from build123d import *

# Parameters (mm, degrees)
BOSS_EXTRUDE1_DEPTH      = 76.2
SKETCH2_W                = 6.985
SKETCH2_H                = 9.525
CUT_EXTRUDE1_DEPTH       = 119.84173867
CUT_EXTRUDE2_DEPTH       = 119.84173867
CUT_EXTRUDE3_DEPTH       = 119.84173867
FILLET1_R                = 2.54
CUT_EXTRUDE4_DEPTH       = 5.08
CUT_EXTRUDE6_DEPTH       = 15.113
FILLET2_R                = 0.508
BOSS_EXTRUDE3_DEPTH      = 31.115
BOSS_EXTRUDE4_DEPTH      = 5.08
CUT_EXTRUDE7_DEPTH       = 85.888967529
CRVPATTERN3_START        = 20.1179377
CRVPATTERN3_OUTLINE_W    = 31.115
CRVPATTERN3_OUTLINE_H    = 7.094089262
CRVPATTERN3_DEPTH        = 4.784345088
CRVPATTERN3_START_2      = 12.248105014
CRVPATTERN3_2_OUTLINE_W  = 31.115
CRVPATTERN3_2_OUTLINE_H  = 6.763167552
CRVPATTERN3_2_DEPTH      = 4.784345087
CRVPATTERN3_START_3      = 4.095774155
CRVPATTERN3_3_OUTLINE_W  = 31.115
CRVPATTERN3_3_OUTLINE_H  = 6.419828923
CRVPATTERN3_3_DEPTH      = 4.784345087
CRVPATTERN3_START_4      = -4.324087509
CRVPATTERN3_4_OUTLINE_W  = 31.115
CRVPATTERN3_4_OUTLINE_H  = 6.064703736
CRVPATTERN3_4_DEPTH      = 4.784345087
CRVPATTERN3_START_5      = 27.690823503
CRVPATTERN3_5_OUTLINE_W  = 31.115
CRVPATTERN3_5_OUTLINE_H  = 6.047255266
CRVPATTERN3_5_DEPTH      = 4.784345088
CRVPATTERN3_START_6      = -12.996021434
CRVPATTERN3_6_OUTLINE_W  = 31.115
CRVPATTERN3_6_OUTLINE_H  = 5.698443985
CRVPATTERN3_6_DEPTH      = 4.784345087
CRVPATTERN3_START_7      = -21.904106282
CRVPATTERN3_7_OUTLINE_W  = 31.115
CRVPATTERN3_7_OUTLINE_H  = 5.321722107
CRVPATTERN3_7_DEPTH      = 4.784345088
CRVPATTERN3_START_8      = -31.031987149
CRVPATTERN3_8_OUTLINE_W  = 31.115
CRVPATTERN3_8_OUTLINE_H  = 4.935229754
CRVPATTERN3_8_DEPTH      = 4.784345087
CRVPATTERN3_START_9      = -40.362905596
CRVPATTERN3_9_OUTLINE_W  = 31.115
CRVPATTERN3_9_OUTLINE_H  = 4.539676505
CRVPATTERN3_9_DEPTH      = 4.784345087
CRVPATTERN3_START_10     = -49.879730415
CRVPATTERN3_10_OUTLINE_W = 31.115
CRVPATTERN3_10_OUTLINE_H = 4.135788586
CRVPATTERN3_10_DEPTH     = 4.784345088
CRVPATTERN3_START_11     = -59.564989077
CRVPATTERN3_11_OUTLINE_W = 31.115
CRVPATTERN3_11_OUTLINE_H = 3.724307516
CRVPATTERN3_11_DEPTH     = 4.784345087
FILLET3_R                = 5.08


# Read off the part's stored shape, not the designer's step: CrvPattern3
with BuildPart() as part:
    # Sketch1 → Boss-Extrude1 (new body)
    with BuildSketch(Plane.XY):
        Polygon((-15.5575, 76.2), (15.5575, 76.2), (15.5575, -76.2), (7.845485509, -76.2), (9.525, -85.725), (-9.525, -85.725), (-7.845485509, -76.2), (-15.5575, -76.2), align=None)
    extrude(amount=BOSS_EXTRUDE1_DEPTH)

    # Sketch2 → Cut-Extrude1 (cut, through all)
    with BuildSketch(Plane(origin=(15.5575, 0, 0), x_dir=(0, 0, -1), z_dir=(1, 0, 0))):
        with Locations((-3.4925, -80.9625)):
            Rectangle(SKETCH2_W, SKETCH2_H)
    extrude(amount=-CUT_EXTRUDE1_DEPTH, mode=Mode.SUBTRACT)

    # Sketch3 → Cut-Extrude2 (cut, through all)
    with BuildSketch(Plane(origin=(15.5575, 0, 0), x_dir=(0, 0, -1), z_dir=(1, 0, 0))):
        with BuildLine():
            Line((-76.2, -85.725), (-76.2, -76.2))
            Line((-76.2, -76.2), (-76.2, 76.2))
            Line((-76.2, 76.2), (-6.541803462, 76.2))
            ThreePointArc((-6.541803462, 76.2), (-58.046669251, 2.411215556), (-76.2, -85.725))
        make_face()
        with BuildLine():
            Line((0, -76.2), (0, 67.75939176))
            ThreePointArc((0, 67.75939176), (-18.20597202, -4.22030412), (0, -76.2))
        make_face()
    extrude(amount=-CUT_EXTRUDE2_DEPTH, mode=Mode.SUBTRACT)

    # Sketch6 → Cut-Extrude3 (cut, through all)
    with BuildSketch(Plane(origin=(15.5575, 0, 0), x_dir=(0, 0, -1), z_dir=(1, 0, 0))):
        with BuildLine():
            ThreePointArc((-28.934409948, -61.883434575), (-23.879909813, -60.517759582), (-22.716254779, -55.412963136))
            ThreePointArc((-22.716254779, -55.412963136), (-30.753414225, -11.294498854), (-26.546552055, 33.352305435))
            ThreePointArc((-26.546552055, 33.352305435), (-49.181053892, -9.446405872), (-61.429710833, -56.286781256))
            ThreePointArc((-61.429710833, -56.286781256), (-59.737369376, -60.827463042), (-55.008021131, -61.883434575))
            ThreePointArc((-55.008021131, -61.883434575), (-41.971215539, -60.062859411), (-28.934409948, -61.883434575))
        make_face()
    extrude(amount=-CUT_EXTRUDE3_DEPTH, mode=Mode.SUBTRACT)

    # Fillet1
    fillet1_edges = [part.edges().sort_by_distance(p)[0] for p in [
        (0, 33.352305435, 26.546552055),
    ]]
    fillet(fillet1_edges, radius=FILLET1_R)

    # Sketch7 → Cut-Extrude4 (cut, symmetric)
    with BuildSketch(Plane(origin=(0, 0, 0), x_dir=(0, 0, -1), z_dir=(1, 0, 0))):
        with BuildLine():
            Line((-30.699128799, 4.016230293), (-17.981752538, 4.016230293))
            ThreePointArc((-17.981752538, 4.016230293), (-17.415803594, -19.667907964), (-13.161921654, -42.973769707))
            Line((-13.161921654, -42.973769707), (-26.264177108, -42.973769707))
            ThreePointArc((-26.264177108, -42.973769707), (-30.179968378, -19.639057999), (-30.699128799, 4.016230293))
        make_face()
    extrude(amount=CUT_EXTRUDE4_DEPTH, both=True, mode=Mode.SUBTRACT)

    # Sketch10 → Cut-Extrude6 (cut, symmetric)
    with BuildSketch(Plane(origin=(15.5575, 76.2, 6.541803462), x_dir=(-1, 0, 0), z_dir=(0, -0.7903999954772005, -0.6125910929401777))):
        Polygon((0, 5.170641427), (6.985, 5.170641427), (0, -3.655858573), align=None)
        Polygon((31.115, 5.170641427), (31.115, -3.655858573), (24.13, 5.170641427), align=None)
    extrude(amount=CUT_EXTRUDE6_DEPTH, both=True, mode=Mode.SUBTRACT)

    # Fillet2
    fillet2_edges = [part.edges().sort_by_distance(p)[0] for p in [
        (0, 76.2, 6.541803462),
        (-14.111333502, 74.930435776, 7.871138317),
        (14.111333502, 74.930435776, 7.871138317),
        (-15.5575, 5.090891194, 56.873019023),
        (15.5575, 5.090891194, 56.873019023),
    ]]
    fillet(fillet2_edges, radius=FILLET2_R)


with BuildPart() as body_2:
    # Sketch11 → Boss-Extrude3 (new body)
    with BuildSketch(Plane(origin=(15.5575, 0, 0), x_dir=(0, 0, -1), z_dir=(1, 0, 0))):
        with BuildLine():
            Line((-8.76443151, 48.407010808), (-3.38019913, 48.407010808))
            ThreePointArc((-3.38019913, 48.407010808), (-7.998658724, -12.530018981), (2.784381833, -72.682972398))
            Line((2.784381833, -72.682972398), (-1.84156903, -72.682972398))
            ThreePointArc((-1.84156903, -72.682972398), (-17.95915827, -12.861548832), (-8.76443151, 48.407010808))
        make_face()
    extrude(amount=-BOSS_EXTRUDE3_DEPTH)


with BuildPart() as body_3:
    # Sketch13 → Boss-Extrude4 (new, symmetric)
    with BuildSketch(Plane(origin=(0, 0, 0), x_dir=(0, 0, -1), z_dir=(1, 0, 0))):
        with BuildLine():
            Line((-13.161921654, -42.973769707), (-26.264177108, -42.973769707))
            ThreePointArc((-26.264177108, -42.973769707), (-30.179968378, -19.639057999), (-30.699128799, 4.016230293))
            Line((-30.699128799, 4.016230293), (-17.981752538, 4.016230293))
            ThreePointArc((-17.981752538, 4.016230293), (-17.415803594, -19.667907964), (-13.161921654, -42.973769707))
        make_face()
    extrude(amount=BOSS_EXTRUDE4_DEPTH, both=True)


with BuildPart() as body_2_1:
    add(body_2.part)

    # Combine1: union body 3
    add(body_3.part)

    # Sketch14 → Cut-Extrude7 (cut, through all)
    with BuildSketch(Plane(origin=(15.5575, 0, 0), x_dir=(0, 0, -1), z_dir=(1, 0, 0))):
        Polygon((-3.636956276, 47.137010808), (-0.743194378, 43.327010808), (-4.923479567, 40.152010808), (-7.817241465, 43.962010808), align=None)
    extrude(amount=-CUT_EXTRUDE7_DEPTH, mode=Mode.SUBTRACT)

    # CrvPattern3 outline → CrvPattern3 (cut)
    with BuildSketch(Plane(origin=(0, 0, 0), x_dir=(1, 0, 0), z_dir=(0, 0.7963472387815729, 0.604839710406786)).offset(CRVPATTERN3_START)):
        with Locations((0, 9.405700103)):
            Rectangle(CRVPATTERN3_OUTLINE_W, CRVPATTERN3_OUTLINE_H)
    extrude(amount=CRVPATTERN3_DEPTH, mode=Mode.SUBTRACT)

    # CrvPattern3 2 outline → CrvPattern3 2 (cut)
    with BuildSketch(Plane(origin=(0, 0, 0), x_dir=(1, 0, 0), z_dir=(0, 0.7963472387815729, 0.604839710406786)).offset(CRVPATTERN3_START_2)):
        with Locations((0, 2.477071696)):
            Rectangle(CRVPATTERN3_2_OUTLINE_W, CRVPATTERN3_2_OUTLINE_H)
    extrude(amount=CRVPATTERN3_2_DEPTH, mode=Mode.SUBTRACT)

    # CrvPattern3 3 outline → CrvPattern3 3 (cut)
    with BuildSketch(Plane(origin=(0, 0, 0), x_dir=(1, 0, 0), z_dir=(0, 0.7963472387815729, 0.604839710406786)).offset(CRVPATTERN3_START_3)):
        with Locations((0, -4.114426542)):
            Rectangle(CRVPATTERN3_3_OUTLINE_W, CRVPATTERN3_3_OUTLINE_H)
    extrude(amount=CRVPATTERN3_3_DEPTH, mode=Mode.SUBTRACT)

    # CrvPattern3 4 outline → CrvPattern3 4 (cut)
    with BuildSketch(Plane(origin=(0, 0, 0), x_dir=(1, 0, 0), z_dir=(0, 0.7963472387815729, 0.604839710406786)).offset(CRVPATTERN3_START_4)):
        with Locations((0, -10.356692871)):
            Rectangle(CRVPATTERN3_4_OUTLINE_W, CRVPATTERN3_4_OUTLINE_H)
    extrude(amount=CRVPATTERN3_4_DEPTH, mode=Mode.SUBTRACT)

    # CrvPattern3 5 outline → CrvPattern3 5 (cut)
    with BuildSketch(Plane(origin=(0, 0, 0), x_dir=(1, 0, 0), z_dir=(0, 0.7963472387815729, 0.604839710406786)).offset(CRVPATTERN3_START_5)):
        with Locations((0, 15.976372367)):
            Rectangle(CRVPATTERN3_5_OUTLINE_W, CRVPATTERN3_5_OUTLINE_H)
    extrude(amount=CRVPATTERN3_5_DEPTH, mode=Mode.SUBTRACT)

    # CrvPattern3 6 outline → CrvPattern3 6 (cut)
    with BuildSketch(Plane(origin=(0, 0, 0), x_dir=(1, 0, 0), z_dir=(0, 0.7963472387815729, 0.604839710406786)).offset(CRVPATTERN3_START_6)):
        with Locations((0, -16.238266732)):
            Rectangle(CRVPATTERN3_6_OUTLINE_W, CRVPATTERN3_6_OUTLINE_H)
    extrude(amount=CRVPATTERN3_6_DEPTH, mode=Mode.SUBTRACT)

    # CrvPattern3 7 outline → CrvPattern3 7 (cut)
    with BuildSketch(Plane(origin=(0, 0, 0), x_dir=(1, 0, 0), z_dir=(0, 0.7963472387815729, 0.604839710406786)).offset(CRVPATTERN3_START_7)):
        with Locations((0, -21.748349778)):
            Rectangle(CRVPATTERN3_7_OUTLINE_W, CRVPATTERN3_7_OUTLINE_H)
    extrude(amount=CRVPATTERN3_7_DEPTH, mode=Mode.SUBTRACT)

    # CrvPattern3 8 outline → CrvPattern3 8 (cut)
    with BuildSketch(Plane(origin=(0, 0, 0), x_dir=(1, 0, 0), z_dir=(0, 0.7963472387815729, 0.604839710406786)).offset(CRVPATTERN3_START_8)):
        with Locations((0, -26.876825708)):
            Rectangle(CRVPATTERN3_8_OUTLINE_W, CRVPATTERN3_8_OUTLINE_H)
    extrude(amount=CRVPATTERN3_8_DEPTH, mode=Mode.SUBTRACT)

    # CrvPattern3 9 outline → CrvPattern3 9 (cut)
    with BuildSketch(Plane(origin=(0, 0, 0), x_dir=(1, 0, 0), z_dir=(0, 0.7963472387815729, 0.604839710406786)).offset(CRVPATTERN3_START_9)):
        with Locations((0, -31.614278838)):
            Rectangle(CRVPATTERN3_9_OUTLINE_W, CRVPATTERN3_9_OUTLINE_H)
    extrude(amount=CRVPATTERN3_9_DEPTH, mode=Mode.SUBTRACT)

    # CrvPattern3 10 outline → CrvPattern3 10 (cut)
    with BuildSketch(Plane(origin=(0, 0, 0), x_dir=(1, 0, 0), z_dir=(0, 0.7963472387815729, 0.604839710406786)).offset(CRVPATTERN3_START_10)):
        with Locations((0, -35.952011383)):
            Rectangle(CRVPATTERN3_10_OUTLINE_W, CRVPATTERN3_10_OUTLINE_H)
    extrude(amount=CRVPATTERN3_10_DEPTH, mode=Mode.SUBTRACT)

    # CrvPattern3 11 outline → CrvPattern3 11 (cut)
    with BuildSketch(Plane(origin=(0, 0, 0), x_dir=(1, 0, 0), z_dir=(0, 0.7963472387815729, 0.604839710406786)).offset(CRVPATTERN3_START_11)):
        with Locations((0, -39.882059434)):
            Rectangle(CRVPATTERN3_11_OUTLINE_W, CRVPATTERN3_11_OUTLINE_H)
    extrude(amount=CRVPATTERN3_11_DEPTH, mode=Mode.SUBTRACT)

    # Fillet3
    fillet3_edges = [body_2_1.edges().sort_by_distance(p)[0] for p in [
        (0, 4.016230293, 30.699128799),
        (0, -42.973769707, 26.264177108),
    ]]
    fillet(fillet3_edges, radius=FILLET3_R)


solid = body_2_1.part
Geometry: final body of the model. Coordinates: model frame, mm. A direction names the side the tool comes from. Round coordinates to 2 decimals unless told otherwise and drop trailing zeros. Write each loop counter-clockwise with the first axis right and the second up, starting at its lowest first coordinate (ties: lowest second). Pieces come first, ordered by that corner, then holes. Notation, with made-up numbers: M 17,80 L 46,80 A7 ccw 46,87 Z; hole C 84.5,54 d10. An arc over 180 degrees is marked long. Write item = value, one per line.
Item 1: Material intervals for line 1 along X through (y, z) = (-21, 24); line 2 along Z through (x, y) = (9.5, -6.5); line 3 along Z through (x, y) = (7.5, -52), sorted ascending. Write a range as [from, to].
Findings:
line_1 = [-5.08, 5.08]
line_2 = [9.32, 18.19]
line_3 = [3.05, 10.47]
Item 2: Section query B-B on z = 14.5. Return loops of the section in (x, y), then the cut area to 3 significant figures.
Findings:
outline = M -15.56,-37.51 L -5.08,-37.51 L -5.08,-42.97 L 5.08,-42.97 L 5.08,-37.51 L 15.56,-37.51 L 15.56,29.07 L -15.56,29.07 Z
area = 2,130 mm^2
Item 3: Section query D-D on y = -64. Return loops of the section in (x, z).
Findings:
outline = M -15.56,-0.24 L 15.56,-0.24 L 15.56,5.9 L -15.56,5.9 Z
Item 4: Section query A-A on y = -15. Return loops of the section in (x, z), then the cut area to 3 significant figures.
Findings:
outline = M -15.56,7.86 L 15.56,7.86 L 15.56,17.82 L 5.08,17.82 L 5.08,30.55 L -5.08,30.55 L -5.08,17.82 L -15.56,17.82 Z
area = 439 mm^2
Item 5: Pull-direction query (Y, two-part tool) for faces 1 (the face through (-0.218, -9.663, 9.474)), 2 (the face through (0, 4.016, 22)), 3 (the face through (-15.558, -12, 12)); classes: pulls with the +Y half, pulls with the -Y half, needs draft (parallel to the pull), parting line crosses it, or undercut.
Findings:
face_1 = undercut
face_2 = pulls with the +Y half
face_3 = needs draft
Item 6: Pin query (flat end, axial travel): P1, Ø12, axis at x = 8.5, z = 12, coming from the -Y side; P2, Ø3, axis at x = -0.5, z = 6.5, coming from the -Y side; P3, Ø1.5, axis at x = -0.5, z = 21.5, coming from the +Y side; P4, Ø3, axis at y = 14.5, z = 20.5, coming from the +X side. Return the tip coordinate at first contact, or that it passes through.
Findings:
P1 = -63.78
P2 = -66.06
P3 = 4.02
P4 = through
Item 7: Access query for faces 4 (the face through (-0.218, -27.54, 7.956)), 5 (the face through (0.218, -65.225, -0.577)). Directions: +Z, -Z, +X, -X, +Y, -Y. A direction counts if a zero-diameter tool reaches every point of the face in a straight line with its end or side. Return the directions, or none.
Findings:
face_4 = -Z, +X, -X
face_5 = -Z, +X, -X, +Y
Item 8: Section query C-C on y = 7. Return loops of the section in (x, z).
Findings:
outline = M -15.56,8.2 L 15.56,8.2 L 15.56,17.79 L -15.56,17.79 Z
